Autodesk Inventor part; units mm, degrees
ref_plane "YZ Plane" through (0, 0, 0) normal (1, 0, 0) x (0, 1, 0)
ref_plane "XZ Plane" through (0, 0, 0) normal (0, 1, 0) x (-1, 0, 0)
ref_plane "XY Plane" through (0, 0, 0) normal (0, 0, 1) x (1, 0, 0)
sketch "Sketch1" plane through (0, 0, 0) normal (0, 0, 1) x (1, 0, 0)
  line L0 (-20, 17.9339) -> (140, 17.9339) construction
  line L1 (-20, 12.9339) -> (140, 12.9339)
  line L2 (140, 22.9339) -> (-20, 22.9339)
  arc A0 (-20, 22.9339) -> (-20, 12.9339) centre (-20, 17.9339) ccw
  arc A1 (140, 12.9339) -> (140, 22.9339) centre (140, 17.9339) ccw
  circle A2 centre (-20, 17.9339) radius 2.5
  circle A3 centre (140, 17.9339) radius 2.5
  circle A4 centre (10, 17.9339) radius 2.5
  line L3 (60, 12.9339) -> (60, -27.0661)
  line L4 (60, -27.0661) -> (20, 12.9339)
  point P0 (0, 0)
  point P1 (60, 17.9339)
  dimension "d0" = 10
  dimension "d1" = 5
  dimension "d2" = 160
  dimension "d7" = 30
  dimension "d10" = 45
  dimension "d11" = 40
  dimension "d12" = 80
extrude "Extrusion1" add sketch "Sketch1" along normal blind 5 contours A0 L2 A1 L1 | A3 | A4
extrude "Extrusion3" cut sketch "Sketch1" along normal up to surface (5 mm away) contours A3 | A4
extrude "Extrusion4" add sketch "Sketch1" along normal up to surface (5 mm away) contours L1 L3 L4
properties material "Copper, Alloy"
Design review of the part built by this model. Coordinates are the model's own, in mm. A direction names the side the tool comes from. Give positions to 0.01 mm unless a question says otherwise; leave off trailing zeros. Write each loop counter-clockwise with the first axis right and the second up, starting at its lowest first coordinate (ties: lowest second). Pieces come first, ordered by that corner, then holes. Notation, with made-up numbers: M 86,-4.5 L 132,-4.5 A18 ccw 132,-0.5 Z; hole C 52.5,87 d4. An arc over 180 degrees is marked long. Answer as a JSON object with one key per item and string values. Group by question number.
1) We need section C-C (y = 0). Give the boundary of the cut face in (x, z), and give its area (3 significant figures).
2) Tool access review of faces 1 (the face through (60, -7, 2)), 2 (the face through (145, 18, 2)): name each direction out of +Z, -Z, +X, -X, +Y, -Y from which nothing blocks a thin tool from reaching the whole face with its end or side.
3) We need section A-A (x = 10). Give the boundary of the cut face in (y, z).
4) Clearance check with flat-ended pins moving along their axes: pin 1 Ø4.5 at (x, y) = (140, 17.93) entering from -Z; pin 2 Ø2.5 at (y, z) = (0, 3) entering from +X; pin 3 Ø1 at (x, z) = (70.5, 0.5) entering from -Y; pin 4 Ø1.5 at (y, z) = (-15.5, 0.5) entering from -X. State where each tip first meets the part, or that it passes through.
5) Mouldability with a two-part tool opening along X and no side actions: class faces 3 (the face through (0, 12.934, 2)), 4 (the face through (142.385, 17.183, 2.465)), 5 (the face through (-25, 18, 2)) as released by +X, released by -X, zero draft, split by the parting line, or undercut.
6) For line 1 along Y through (x, z) = (140, 1.3); line 2 along X through (y, z) = (16, 3.4); line 3 along X through (y, z) = (20, 1.85), list the stretches that pass through material, from the lowest coordinate up.
7) We need section B-B (z = 3.25). Give the boundary of the cut face in (x, y), and give its area (3 significant figures).
Answer key:
{
 "1": {"outline": "M 32.93,0 L 60,0 L 60,5 L 32.93,5 Z", "area": "135 mm²"},
 "2": {"face 1": "+Z, -Z, +X, -Y", "face 2": "+Z, -Z, +X"},
 "3": {"outline": "M 12.93,0 L 15.43,0 L 15.43,5 L 12.93,5 Z; M 20.43,0 L 22.93,0 L 22.93,5 L 20.43,5 Z"},
 "4": {"pin 1": "passes through", "pin 2": "stops at x = 60", "pin 3": "stops at y = 12.93", "pin 4": "stops at x = 47.68"},
 "5": {"face 3": "zero draft", "face 4": "undercut", "face 5": "released by -X"},
 "6": {"line 1": "y = 12.93 to 15.43, 20.43 to 22.93", "line 2": "x = -24.61 to -21.58, -18.42 to 8.42, 11.58 to 138.42, 141.58 to 144.61", "line 3": "x = -24.55 to -21.41, -18.59 to 8.59, 11.41 to 138.59, 141.41 to 144.55"},
 "7": {"outline": "M -20,12.93 L 20,12.93 L 60,-27.07 L 60,12.93 L 140,12.93 A5 ccw 140,22.93 L -20,22.93 A5 ccw Z; hole C -20,17.93 d5; hole C 10,17.93 d5; hole C 140,17.93 d5", "area": "2,420 mm²"}
}
